from build123d import *

# Parameters (mm, degrees)
BOSS_EXTRUDE1_DEPTH = 100
SKETCH5_OUTSIDE_W   = 62.398
SKETCH5_OUTSIDE_H   = 242.398
CUT_EXTRUDE1_DEPTH  = 21


with BuildPart() as part:
    # Sketch4 → Boss-Extrude1 (new body, symmetric)
    with BuildSketch(Plane.XY):
        with BuildLine():
            Line((3, -10), (8.25, -10))
            ThreePointArc((8.25, -10), (9.487436867, -9.487436867), (10, -8.25))
            Line((10, -8.25), (10, -3))
            ThreePointArc((10, -3), (9.853553391, -2.646446609), (9.5, -2.5))
            Line((9.5, -2.5), (8.424621202, -2.5))
            ThreePointArc((8.424621202, -2.5), (8.071067812, -2.646446609), (7.924621202, -3))
            Line((7.924621202, -3), (7.924621202, -5.25))
            ThreePointArc((7.924621202, -5.25), (7.615962919, -5.711939766), (7.071067812, -5.603553391))
            Line((7.071067812, -5.603553391), (4.478679656, -3.011165235))
            ThreePointArc((4.478679656, -3.011165235), (3.828361402, -2.037895189), (3.6, -0.889844892))
            Line((3.6, -0.889844892), (3.6, 0))
            Line((3.6, 0), (2.15, 0))
            ThreePointArc((2.15, 0), (1.52027958, -1.52027958), (0, -2.15))
            Line((0, -2.15), (0, -3.6))
            Line((0, -3.6), (0.889844892, -3.6))
            ThreePointArc((0.889844892, -3.6), (2.037895189, -3.828361402), (3.011165235, -4.478679656))
            Line((3.011165235, -4.478679656), (5.603553391, -7.071067812))
            ThreePointArc((5.603553391, -7.071067812), (5.711939766, -7.615962919), (5.25, -7.924621202))
            Line((5.25, -7.924621202), (3, -7.924621202))
            ThreePointArc((3, -7.924621202), (2.646446609, -8.071067812), (2.5, -8.424621202))
            Line((2.5, -8.424621202), (2.5, -9.5))
            ThreePointArc((2.5, -9.5), (2.646446609, -9.853553391), (3, -10))
        make_face()
    extrude(amount=BOSS_EXTRUDE1_DEPTH, both=True)

    # Mirror1: part across plane


with BuildPart() as part_1:
    add(part.part)
    add(part.part.mirror(Plane(origin=(0, 0, 0), x_dir=(0, 0, 1), z_dir=(1, 0, 0))))

    # Mirror2: part across plane


with BuildPart() as part_2:
    add(part_1.part)
    add(part_1.part.mirror(Plane.ZX))

    # Sketch5 outside → Cut-Extrude1 (cut, through all)
    with BuildSketch(Plane(origin=(0, 10, 0), x_dir=(1, 0, 0), z_dir=(0, 1, 0))):
        Rectangle(SKETCH5_OUTSIDE_W, SKETCH5_OUTSIDE_H)
        Polygon((-10, -100), (62, 24.707658145), (-11.612159322, 67.207658145), align=None, mode=Mode.SUBTRACT)
    extrude(amount=-CUT_EXTRUDE1_DEPTH, mode=Mode.SUBTRACT)


solid = part_2.part
Design review of the part built by this model. Coordinates are the model's own, in mm. A direction names the side the tool comes from. Coordinates: 2 decimals unless noted, no trailing zeros. One line per item, written item: value.
1) Clearance check with flat-ended pins moving along their axes: P1, Ø8, axis at x = -2.5, y = 4.5, coming from the -Z side; P2, Ø0.9, axis at y = 9, z = 16, coming from the +X side; P3, Ø0.5, axis at x = 9, z = 24.5, coming from the +Y side; P4, Ø4, axis at y = 2.5, z = 76, coming from the -X side. State where each tip first meets the part, or that it passes through.
Output values:
P1: stops at z = -64.24
P2: stops at x = 9.97
P3: stops at y = 9.93
P4: stops at x = -10
2) Draft analysis for pull direction Y (two halves, no side actions). For faces 3 (the face through (4.29, -5.76, 10.3)), 4 (the face through (6, 10, 10)), 5 (the face through (10, 6, 6)), 6 (the face through (-5.793, -4.326, 16.287)), state which applies: +Y half, -Y half, draft (parallel to the pull), parting line (faces both ways), or undercut.
Output values:
face 3: undercut
face 4: +Y half
face 5: draft
face 6: undercut
3) Machinability: for faces 1 (the face through (-6, 10, 17)), 2 (the face through (-5.793, 4.326, 16.287)), which of the approach directions +Z, -Z, +X, -X, +Y, -Y give a long, thin tool a straight path to every point of the face, cutting with its end or side? Answer none if there is none.
Output values:
face 1: +Z, -Z, +X, -X, +Y
face 2: +Z, -Z
4) To check wall thickness, follow probe 1 along Y at (x, z) = (3, -7.5); probe 2 along X at (y, z) = (-5.25, 34). State the ranges of each line that lie inside material, in increasing order. Write a range as [from, to].
Output values:
probe 1: y = [-10, -7.92], [-4.47, 4.47], [7.92, 10]
probe 2: x = [-10, -7.92], [-6.72, -3.78], [3.78, 6.72], [7.92, 10]
